For this review, use the dimensioned drawing (mm, ordinates from the lowest corner) and the shaded views. A direction names the side the tool comes from. Coordinates: 2 decimals unless noted, no trailing zeros. Order: outer loops, then holes, each group sorted by start corner. A loop starts at its lowest first (then second) coordinate and runs counter-clockwise, first axis right, second up. Notation, with made-up numbers: M 5.25,70.25 L 32.25,70.25 A25 ccw 32.25,102.25 Z; hole C 40,27.5 d8. An arc over 180 degrees is marked long. Answer in a Markdown table with one row per item.
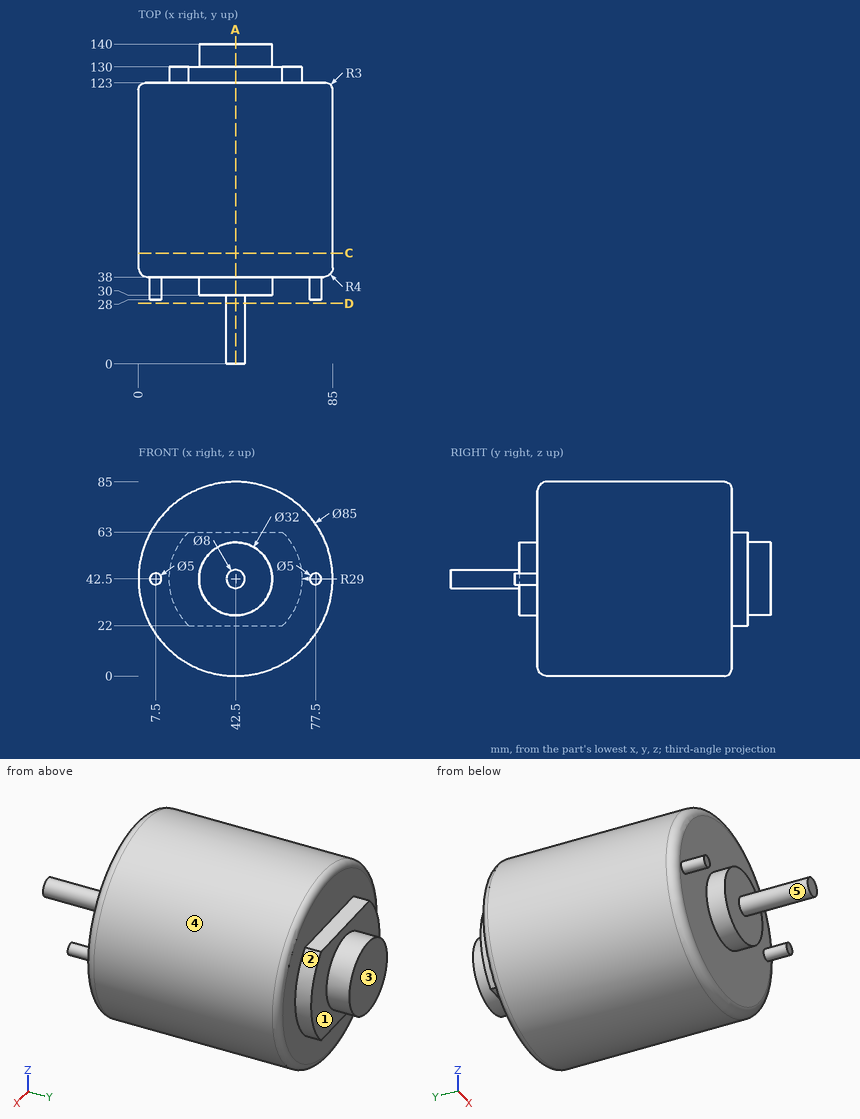
(1) Insertion check: pin 1 Ø2 at (y, z) = (44, 64) entering from -X; pin 2 Ø5.5 at (x, y) = (42.5, 126.5) entering from +Z; pin 3 Ø4 at (x, z) = (6.5, 42.5) entering from -Y. Each pin has a flat end and moves straight along its axis. Give the tip position at first contact, or say it passes through.
Return value:
| item | result |
|---|---|
| pin 1 | stops at x = 5.27 |
| pin 2 | stops at z = 63 |
| pin 3 | stops at y = 28 |
(2) For the marked faces 1, 2, 3, 4 and 5, list the 3-axis set-ups (+Z, -Z, +X, -X, +Y, -Y) from which the entire face can be reached by the end or side of a thin tool; tool diameter is ignored.
Return value:
| item | result |
|---|---|
| face 1 | +Y |
| face 2 | +X, +Y |
| face 3 | +Z, -Z, +X, -X, +Y |
| face 4 | +Y, -Y |
| face 5 | -Y |
(3) Add section A-A, the plane x = 42.5. Give the boundary of the cut face in (y, z).
Return value:
| item | result |
|---|---|
| outline | M 0,38.5 L 30,38.5 L 30,26.5 L 38,26.5 L 38,4 A4 ccw 42,0 L 120,0 A3 ccw 123,3 L 123,22 L 130,22 L 130,26.5 L 140,26.5 L 140,58.5 L 130,58.5 L 130,63 L 123,63 L 123,82 A3 ccw 120,85 L 42,85 A4 ccw 38,81 L 38,58.5 L 30,58.5 L 30,46.5 L 0,46.5 Z |
(4) For line 1 along Y through (x, z) = (24, 30); line 2 along Y through (x, z) = (16.5, 67); line 3 along Z through (x, y) = (51.5, 124), list the stretches that pass through material, from the lowest coordinate up. Write a range as from..to.
Return value:
| item | result |
|---|---|
| line 1 | y = 38..130 |
| line 2 | y = 38..123 |
| line 3 | z = 22..63 |
(5) Add section C-C, the plane y = 48.5. Give the boundary of the cut face in (x, z), and give its area (3 significant figures).
Return value:
| item | result |
|---|---|
| outline | C 42.5,42.5 d85 |
| area | 5,670 mm2 |
(6) Add section D-D, the plane y = 26.5. Give the boundary of the cut face in (x, z).
Return value:
| item | result |
|---|---|
| outline | C 42.5,42.5 d8 |
